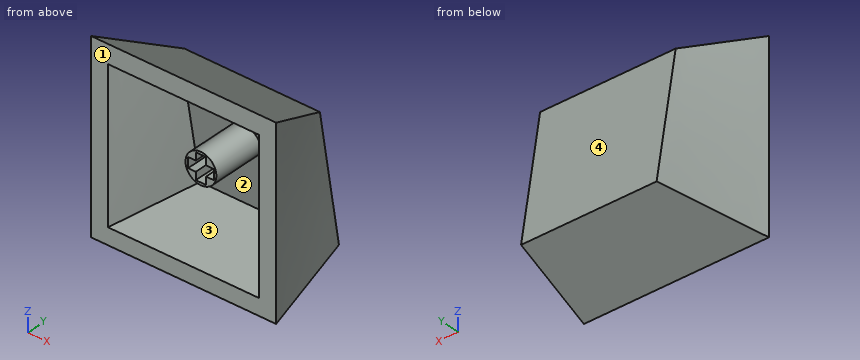
```python
from build123d import *

# Parameters (mm, degrees)
SHELL1_T            = -1.6
BOSS_EXTRUDE1_REACH = 20.248
BOSS_EXTRUDE1_START = -2
SKETCH4_R           = 1.5
CUT_EXTRUDE1_REACH  = 17.087
SKETCH5_W           = 0.75
SKETCH5_H           = 1
SKETCH5_W_2         = 1
SKETCH5_H_2         = 0.75


with BuildPart() as part:
    # Sketch1 → Loft1 section 0
    with BuildSketch(Plane(origin=(0, 0, 0), x_dir=(1, 0, 0), z_dir=(0, 1, 0))):
        with BuildLine():
            Line((-9, 9), (9, 9))
            Line((9, 9), (9, -9))
            Line((9, -9), (-9, -9))
            Line((-9, -9), (-9, 9))
        make_face()
    # Sketch3 → Loft1 section 1
    with BuildSketch(Plane(origin=(0, 8.483501929, 1.435669557), x_dir=(0, 0.16685830369290802, -0.9859808854580931), z_dir=(0, 0.9859808854580931, 0.16685830369290802))):
        with BuildLine():
            Line((-3.496990657, 6.59241989), (9.687849122, 6.59241989))
            Line((9.687849122, 6.59241989), (9.687849122, -6.59241989))
            Line((9.687849122, -6.59241989), (-3.496990657, -6.59241989))
            Line((-3.496990657, -6.59241989), (-3.496990657, 6.59241989))
        make_face()
    loft()

    # Shell1
    shell1_openings = [part.faces().sort_by_distance(p)[0] for p in [
        (0, 0, 0),
    ]]
    offset(amount=SHELL1_T, openings=shell1_openings, kind=Kind.INTERSECTION)

    # Boss-Extrude1: up to this plane
    boss_extrude1_end = Plane(origin=(0, 6.905932512, 1.168696271), z_dir=(0, 0.9859808854580933, 0.16685830369290802))
    # Sketch4 → Boss-Extrude1 (add, up to the surface)
    with BuildSketch(Plane.XZ.offset(BOSS_EXTRUDE1_START), mode=Mode.PRIVATE) as boss_extrude1_sk1:
        with Locations(Location((0, 0, 0), (0, 0, 270))):
            Circle(SKETCH4_R)
    boss_extrude1_tool1 = split(extrude(boss_extrude1_sk1.sketch, amount=-BOSS_EXTRUDE1_REACH, mode=Mode.PRIVATE), bisect_by=boss_extrude1_end, keep=Keep.BOTH, mode=Mode.PRIVATE)
    add(boss_extrude1_tool1.solids().sort_by_distance((0, 2, 0))[0])

    # Cut-Extrude1: up to this plane
    cut_extrude1_end = Plane(origin=(0, 6.41294207, 1.085267119), z_dir=(0, 0.9859808854580933, 0.16685830369290802))
    # Sketch5 → Cut-Extrude1 (cut, up to the surface)
    with BuildSketch(Plane.XZ.offset(-2), mode=Mode.PRIVATE) as cut_extrude1_sk1:
        with Locations((-0.875, 0)):
            Rectangle(SKETCH5_W, SKETCH5_H)
    cut_extrude1_tool1 = split(extrude(cut_extrude1_sk1.sketch, amount=-CUT_EXTRUDE1_REACH, mode=Mode.PRIVATE), bisect_by=cut_extrude1_end, keep=Keep.BOTH, mode=Mode.PRIVATE)
    add(cut_extrude1_tool1.solids().sort_by_distance((-0.875, 2, 0))[0], mode=Mode.SUBTRACT)
    # Sketch5 → Cut-Extrude1 (cut, up to the surface)
    with BuildSketch(Plane.XZ.offset(-2), mode=Mode.PRIVATE) as cut_extrude1_sk2:
        Rectangle(SKETCH5_W_2, SKETCH5_H)
    cut_extrude1_tool2 = split(extrude(cut_extrude1_sk2.sketch, amount=-CUT_EXTRUDE1_REACH, mode=Mode.PRIVATE), bisect_by=cut_extrude1_end, keep=Keep.BOTH, mode=Mode.PRIVATE)
    add(cut_extrude1_tool2.solids().sort_by_distance((0, 2, 0))[0], mode=Mode.SUBTRACT)
    # Sketch5 → Cut-Extrude1 (cut, up to the surface)
    with BuildSketch(Plane.XZ.offset(-2), mode=Mode.PRIVATE) as cut_extrude1_sk3:
        with Locations((0, 0.875)):
            Rectangle(SKETCH5_W_2, SKETCH5_H_2)
    cut_extrude1_tool3 = split(extrude(cut_extrude1_sk3.sketch, amount=-CUT_EXTRUDE1_REACH, mode=Mode.PRIVATE), bisect_by=cut_extrude1_end, keep=Keep.BOTH, mode=Mode.PRIVATE)
    add(cut_extrude1_tool3.solids().sort_by_distance((0, 2, 0.875))[0], mode=Mode.SUBTRACT)
    # Sketch5 → Cut-Extrude1 (cut, up to the surface)
    with BuildSketch(Plane.XZ.offset(-2), mode=Mode.PRIVATE) as cut_extrude1_sk4:
        with Locations((0.875, 0)):
            Rectangle(SKETCH5_W, SKETCH5_H)
    cut_extrude1_tool4 = split(extrude(cut_extrude1_sk4.sketch, amount=-CUT_EXTRUDE1_REACH, mode=Mode.PRIVATE), bisect_by=cut_extrude1_end, keep=Keep.BOTH, mode=Mode.PRIVATE)
    add(cut_extrude1_tool4.solids().sort_by_distance((0.875, 2, 0))[0], mode=Mode.SUBTRACT)
    # Sketch5 → Cut-Extrude1 (cut, up to the surface)
    with BuildSketch(Plane.XZ.offset(-2), mode=Mode.PRIVATE) as cut_extrude1_sk5:
        with Locations((0, -0.875)):
            Rectangle(SKETCH5_W_2, SKETCH5_H_2)
    cut_extrude1_tool5 = split(extrude(cut_extrude1_sk5.sketch, amount=-CUT_EXTRUDE1_REACH, mode=Mode.PRIVATE), bisect_by=cut_extrude1_end, keep=Keep.BOTH, mode=Mode.PRIVATE)
    add(cut_extrude1_tool5.solids().sort_by_distance((0, 2, -0.875))[0], mode=Mode.SUBTRACT)


solid = part.part
```
Can you work these out from the model? Positions are in its coordinate system, mm. Face numbers are marked on the shaded views. A direction names the side the tool comes from. Give positions to 0.01 mm unless a question says otherwise; leave off trailing zeros. Use CSV: the item, a comma, the result in double quotes. Start each with the question number.
1. On a 3-axis mill with a long thin cutter (end or side, diameter ignored), from which of +Z, -Z, +X, -X, +Y, -Y can I reach the whole of each face in a straight line? I mean the marked faces 1 and 2. Say none if no direction works.
2. For P1, Ø1, axis at y = 8.5, z = -1, coming from the +X side; P2, Ø0.6, axis at x = 1, y = 3.5, coming from the -Z side; P3, Ø3.5, axis at x = 0, z = 0, coming from the -Y side, each with a flat end and sliding along its axis, tell me the tip position at first contact or that it passes through.
3. Imagine slicing it at A-A, the plane y = 2.25. Count the separate pieces of the cut face and the enclosed holes in it, plus the area to 3 significant figures.
4. If we mould it in two halves opening along X, with no side actions, what happens to the marked faces 3 and 4? For each: released by +X, released by -X, zero draft, split by the parting line, or undercut.
5. If I drill on L1, parallel to X at y = 0.5, z = -5.5; L2, parallel to X at y = 4, z = 0.25; L3, parallel to Z at x = -4, y = 3, over which ranges is the centre line in solid material (lowest first)?
Response values:
1,face 1,"+Z, -Z, +X, -X, -Y"
1,face 2,"-Y"
2,P1,"x = 6.84"
2,P2,"z = -8.72"
2,P3,"y = 2"
3,separate pieces,"2"
3,enclosed holes,"2"
3,area,"104 mm^2"
4,face 3,"undercut"
4,face 4,"zero draft"
5,L1,"-8.88 to -7.23, 7.23 to 8.88"
5,L2,"-7.91 to -6.25, -1.48 to -1.25, 1.25 to 1.48, 6.25 to 7.91"
5,L3,"-8.74 to -7.13, 5.63 to 7.44"
